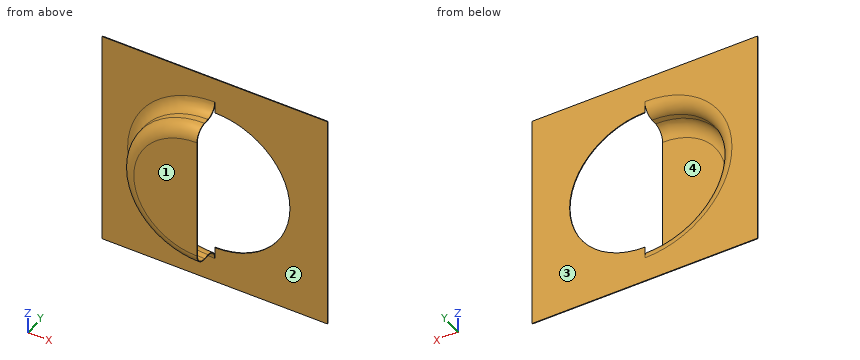
Autodesk Inventor part; units mm, degrees
ref_plane "Work Plane1" through (75, 0.5, -75) normal (0, 0, -1) x (-1, 0, 0)
ref_plane "YZ Plane" through (0, 0, 0) normal (1, 0, 0) x (0, 1, 0)
ref_plane "XZ Plane" through (0, 0, 0) normal (0, 1, 0) x (-1, 0, 0)
sketch "Sketch1" plane through (0, 0, 0) normal (0, 1, 0) x (-1, 0, 0)
  line L0 (0, 0) -> (-150, 0)
  line L1 (-150, 0) -> (-150, -150)
  line L2 (-150, -150) -> (0, -150)
  line L3 (0, -150) -> (0, 0)
  dimension "d0" = 150
  dimension "d1" = 150
extrude "Plate1" add sketch "Sketch1" along normal blind 0.5
sketch "Sketch2" plane through (0, 0.5, 0) normal (0, 1, 0) x (1, 0, 0)
  arc A0 (75, 133) -> (75, 17) centre (75, 75) ccw
  line L0 (0, 0) -> (0, 150)
  line L1 (0, 150) -> (150, 150)
  line L2 (75, 17) -> (75, 133) construction
  arc A1 (75, 25) -> (75, 125) centre (75, 75) ccw
  line L3 (75, 125) -> (75, 133)
  line L4 (75, 25) -> (75, 17)
  arc A2 (75, 17) -> (75, 133) centre (75, 75) ccw construction
  dimension "d3" = 75
  dimension "d4" = 75
  dimension "d5" = 116
  dimension "d7" = 50
extrude "Extrusion1" cut sketch "Sketch2" against normal blind 0.5
ref_plane "Work Plane1" through (75, 0.5, -75) normal (0, 0, -1) x (-1, 0, 0)
sketch "Sketch3" plane through (75, 0.5, -75) normal (0, 0, -1) x (-1, 0, 0)
  line L0 (58, 0) -> (0, 0) construction
  line L1 (0, 0) -> (0, -0.5)
  line L2 (0, 0) -> (0, -20)
  line L3 (0, -20) -> (42, -20)
  arc A0 (42, -20) -> (50, -12) centre (42, -12) ccw
  line L4 (50, -12) -> (50, -8)
  arc A1 (58, 0) -> (50, -8) centre (58, -8) ccw
  line L5 (58, 0) -> (58, -0.5)
  arc A2 (58, -0.5) -> (50.5, -8) centre (58, -8) ccw
  line L6 (50.5, -8) -> (50.5, -12)
  arc A3 (42, -20.5) -> (50.5, -12) centre (42, -12) ccw
  line L7 (42, -20.5) -> (0, -20.5)
  line L8 (0, -20.5) -> (0, -20)
  line L9 (42, -20) -> (42, -20.5) construction
  line L10 (50.5, -8) -> (50, -8) construction
  point P0 (75, -0.5)
  dimension "d10" = 20
  dimension "d12" = 8
  dimension "d13" = 8
  dimension "d14" = 0.5
  dimension "d15" = 0.5
  dimension "d16" = 0.5
revolve "Revolution1" add sketch "Sketch3" angle 180 mid plane about axis through (75, 0.5, -75) along (0, -1, 0)
equation "\"d8\" = Thickness"
equation "\"d14\" = Thickness"
equation "\"d15\" = Thickness"
equation "\"d16\" = Thickness"
equation "\"d2\" = Thickness"
equation "\"BendRadius\" = Thickness"
equation "\"BendReliefWidth\" = Thickness"
equation "\"BendReliefDepth\" = 0.5 * Thickness"
equation "\"CornerReliefSize\" = 4 * Thickness"
equation "\"MinimumRemnant\" = 2 * Thickness"
equation "\"TransitionRadius\" = BendRadius"
equation "\"JacobiRadiusSize\" = BendRadius"
equation "\"GapSize\" = Thickness"
properties part number "A3.2"
CAD build for the part. Positions are in the model's coordinates, mm. Face numbers are marked on the shaded views. A direction names the side the tool comes from. Round coordinates to 2 decimals unless told otherwise and drop trailing zeros. Write each loop counter-clockwise with the first axis right and the second up, starting at its lowest first coordinate (ties: lowest second). Pieces come first, ordered by that corner, then holes. Notation, with made-up numbers: (59, 17.5) - (76, 17.5) arc R8 cw to (76, 24.5) - close; hole circle Ø6 at (67, 69). An arc over 180 degrees is marked (long way). Write item = value, one per line. Start each with the question number.
Q1. Band-saw the part on B-B (x = 117). Give the cut face in (y, z), then the cut area to 3 significant figures.
Q2. Drop flat-ended pins along their axis: pin 1 (6 mm diameter, centred on y = -12.5, z = -54, fed in from +X); pin 2 (3 mm diameter, centred on y = -14, z = -116.5, fed in from +X); pin 3 (2 mm diameter, centred on y = -5, z = -21, fed in from +X); pin 4 (1.5 mm diameter, centred on y = -11, z = -101.5, fed in from +X). Give the stop position or say it passes through.
Q3. Which spindle directions (+Z, -Z, +X, -X, +Y, -Y) get a long thin tool onto all of the face, cutting with end or side? Do the marked faces 1 and 2. Say none if no direction does.
Q4. Mould opens along Z. For the marked faces 3 and 4 say: pulls with the +Z half, pulls with the -Z half, needs draft (parallel to the pull), parting line crosses it, or undercut.
Q5. Band-saw the part on C-C (z = -138.5). Give the cut face in (x, y), then the cut area to 3 significant figures.
Q6. Probe L1, parallel to Y at x = 133.5, z = -108; L2, parallel to Z at x = 42, y = -3.25; L3, parallel to Y at x = 39, z = -56.5. List the from-to ranges inside material, lowest first. Write a range as from..to.
Q7. Band-saw the part on A-A (z = -75). Give the cut face in (x, y).
Q8. Band-saw the part on D-D (x = 14). Give the cut face in (y, z), then the cut area to 3 significant figures.
Answers below:
q1.outline = (0, -150) - (0.5, -150) - (0.5, -102.13) - (0, -102.13) - close; (0, -47.87) - (0.5, -47.87) - (0.5, 0) - (0, 0) - close
q1.area = 47.9 mm2
q2.pin_1 = 31.39
q2.pin_2 = 50.52
q2.pin_3 = through
q2.pin_4 = 33.08
q3.face_1 = +Z, -Z, +X, -X, -Y
q3.face_2 = -Y
q4.face_3 = needs draft
q4.face_4 = undercut
q5.outline = (0, 0) - (150, 0) - (150, 0.5) - (0, 0.5) - close
q5.area = 75.0 mm2
q6.L1 = 0..0.5
q6.L2 = -114.95..-114.18, -35.82..-35.05
q6.L3 = -20..-19.5
q7.outline = (0, 0) - (17, 0) arc R7.5 cw to (24.5, -7.5) - (24.5, -11.5) arc R8.5 ccw to (33, -20) - (75, -20) - (75, -19.5) - (33, -19.5) arc R8 cw to (25, -11.5) - (25, -7.5) arc R8 ccw to (17, 0.5) - (0, 0.5) - close; (125, 0) - (150, 0) - (150, 0.5) - (125, 0.5) - close
q8.outline = (0, -150) - (0.5, -150) - (0.5, 0) - (0, 0) - close
q8.area = 75.0 mm2
